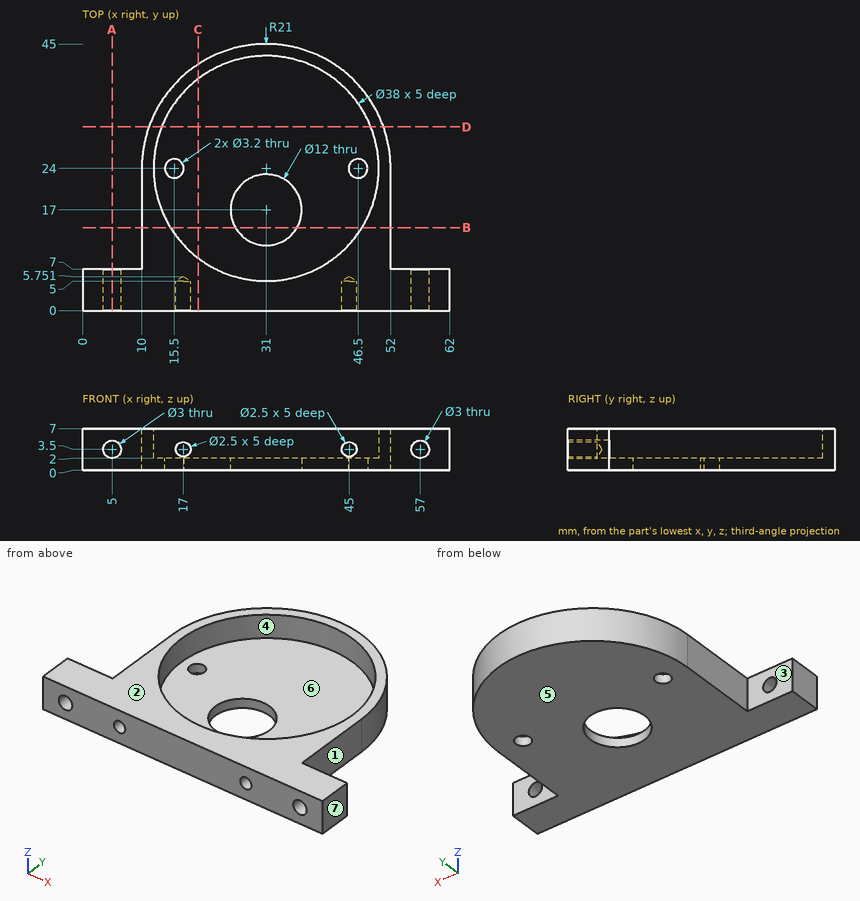
Answer from the drawing. Dimensions are ordinates in mm from the lowest x, y and z of the part. A direction names the side the tool comes from. Round coordinates to 2 decimals unless told otherwise and drop trailing zeros. Write each loop counter-clockwise with the first axis right and the second up, starting at its lowest first coordinate (ties: lowest second). Pieces come first, ordered by that corner, then holes. Notation, with made-up numbers: (36.25, -21.75) -> (51.25, -21.75) arc R16 ccw to (51.25, -2.75) -> close; hole circle Ø9 at (72.5, 34.25). An arc over 180 degrees is marked (long way). Answer in a Markdown table with one row per item. Add a question column.
1) Find section B-B, the plane y = 14. Determine the outline of the cut face in (x, z), and give its area (3 significant figures).
2) Find section C-C, the plane x = 19.5. Determine the outline of the cut face in (y, z).
3) Find section A-A, the plane x = 5. Determine the outline of the cut face in (y, z), and give its area (3 significant figures).
4) Which of the six approach directions +Z, -Z, +X, -X, +Y, -Y give full straight-line access (tool end or side, diameter ignored) to the marked faces 1, 2 and 3?
5) Find section D-D, the plane y = 31. Determine the outline of the cut face in (x, z).
6) Determine the mould class of the marked faces 4, 5, 6 and 7 for opening direction X: pulls with the +X half, pulls with the -X half, needs draft (parallel to the pull), parting line crosses it, or undercut.
7) Given P1, Ø19, axis at x = 22.5, y = 25.5, coming from the +Z side; P2, Ø4, axis at y = 34.5, z = 2, coming from the -X side; P3, Ø2, axis at x = 57.5, z = 2.5, coming from the +Y side, each flat-ended and moving along its own axis, determine where each tip first touches the part or whether it passes through.
8) Consider line 1 (X direction, y = 2.75, z = 3.5); line 2 (Y direction, x = 31, z = 5.8); line 3 (Z direction, x = 14, y = 17). Determine where each line is inside the solid, lowest interval first.
Findings below:
| question | item | result |
|---|---|---|
| 1 | outline | (10, 0) -> (25.8, 0) -> (25.8, 2) -> (14.84, 2) -> (14.84, 7) -> (10, 7) -> close; (36.2, 0) -> (52, 0) -> (52, 7) -> (47.16, 7) -> (47.16, 2) -> (36.2, 2) -> close |
| 1 | area | 112 mm² |
| 2 | outline | (0, 0) -> (41.57, 0) -> (41.57, 7) -> (39.12, 7) -> (39.12, 2) -> (8.88, 2) -> (8.88, 7) -> (0, 7) -> close |
| 3 | outline | (0, 0) -> (7, 0) -> (7, 2) -> (0, 2) -> close; (0, 5) -> (7, 5) -> (7, 7) -> (0, 7) -> close |
| 3 | area | 28.0 mm² |
| 4 | face 1 | +Z, -Z, +X, +Y |
| 4 | face 2 | +Z, +X, -X, +Y, -Y |
| 4 | face 3 | +Z, -Z, -X, +Y |
| 5 | outline | (11.2, 0) -> (50.8, 0) -> (50.8, 7) -> (48.66, 7) -> (48.66, 2) -> (13.34, 2) -> (13.34, 7) -> (11.2, 7) -> close |
| 6 | face 4 | undercut |
| 6 | face 5 | needs draft |
| 6 | face 6 | undercut |
| 6 | face 7 | pulls with the +X half |
| 7 | P1 | z = 2 |
| 7 | P2 | x = 11.8 |
| 7 | P3 | y = 7 |
| 8 | line 1 | 0 to 3.5, 6.5 to 15.75, 18.25 to 43.75, 46.25 to 55.5, 58.5 to 62 |
| 8 | line 2 | 0 to 5, 43 to 45 |
| 8 | line 3 | 0 to 2 |
